For this review, take the finished solid that the model builds, in its own axes (mm). Round coordinates to 2 decimals unless told otherwise and drop trailing zeros. Loops run counter-clockwise (first coordinate to the right, second up) from the corner with the lowest first, then second, coordinate; pieces in that order, holes last. Notation, with made-up numbers: (88.25, -28.75) -> (106.25, -28.75) arc R19 ccw to (106.25, -13.75) -> close; hole circle Ø2 at (21, 61.5). An arc over 180 degrees is marked (long way). One line per question, with ' | ' between items. Start each with the question number.
1. Consider section C-C (y = -9). Write out the cut boundary in (x, z) (3 decimals).
2. Wall thickness on line 1 along X through (y, z) = (-5.75, 9.5); line 2 along Z through (x, y) = (-19.5, -0.5); line 3 along X through (y, z) = (-2.75, 5.5): over which ranges is each line inside the solid? List them lowest first.
3. For pin 1 Ø5 at (x, y) = (20.5, -8.5) entering from -Z, flat-tipped, find the tip position at first contact; note if it passes through.
4. Draft analysis for pull direction X (two halves, no side actions). For faces 1 (the face through (14, -4, 19.05)), 2 (the face through (47.722, -5, 9)), 3 (the face through (-25.36, -4.36, 2.69)), 4 (the face through (-23.99, -4.63, 5.66)), state which applies: pulls with the +X half, pulls with the -X half, needs draft (parallel to the pull), parting line crosses it, or undercut.
5. Consider section B-B (x = -21). Write out the cut boundary in (y, z), and give its area (3 significant figures).
6. Consider section A-A (z = 10.5). Write out the cut boundary in (x, y).
7. Consider section D-D (z = 17). Write out the cut boundary in (x, y), and give its area (3 significant figures).
```python
from build123d import *

# Parameters (mm, degrees)
F0_W        = 76.2
F0_H        = 19.05
F1_DEPTH    = 19.05
F3_D        = 12.7
F4_T1_DEPTH = 68.58


# Not quite as in the source:
# - a fillet or chamfer that OpenCascade refuses, or shapes differently, is made with other operations: its cross-section is extruded or revolved along the edge and cut away or added


with BuildPart() as f1:
    # F0 (on Top) → F1 (new body)
    with BuildSketch(Plane.XY):
        with Locations((9.6218887268, -4.4917178258)):
            Rectangle(F0_W, F0_H)
    extrude(amount=F1_DEPTH)

    # F3 (through all)
    with Locations(Plane(origin=(0, 5.0332821742, 0), x_dir=(-1, 0, 0), z_dir=(0, 1, 0))):
        with Locations((18.9531112732, 9.525)):
            Hole(F3_D / 2)

    # F4: fillet of radius 9.906 on 2 edges, made by hand

    # F4_s2 → F4_t1 (cut)
    with BuildSketch(Plane.XZ.offset(-29.7982821742)):
        with BuildLine():
            ThreePointArc((-18.5721112732, 19.05), (-25.5767110476, 16.1485997744), (-28.4781112732, 9.144))
            Line((-28.4781112732, 9.144), (-28.4781112732, 19.05))
            Line((-28.4781112732, 19.05), (-18.5721112732, 19.05))
        make_face()
        with BuildLine():
            ThreePointArc((-18.5721112732, 0), (-25.5767110476, 2.9014002256), (-28.4781112732, 9.906))
            Line((-28.4781112732, 9.906), (-28.4781112732, 0))
            Line((-28.4781112732, 0), (-18.5721112732, 0))
        make_face()
    extrude(amount=F4_T1_DEPTH, mode=Mode.SUBTRACT)


solid = f1.part
```
Answer block:
1) outline: (-28.471, 9.525) arc R9.906 ccw to (-18.572, 0) -> (47.722, 0) -> (47.722, 19.05) -> (-18.572, 19.05) arc R9.906 ccw to start; hole circle Ø12.7 at (-18.953, 9.525)
2) line 1: x = -28.47 to -25.3, -12.6 to 47.72 | line 2: z = 0.04 to 3.2, 15.85 to 19.01 | line 3: x = -27.44 to -23.86, -14.04 to 47.72
3) pin 1: stops at z = 0
4) face 1: needs draft | face 2: pulls with the +X half | face 3: pulls with the -X half | face 4: undercut
5) outline: (-14.02, 0.3) -> (5.03, 0.3) -> (5.03, 3.51) -> (-14.02, 3.51) -> close; (-14.02, 15.54) -> (5.03, 15.54) -> (5.03, 18.75) -> (-14.02, 18.75) -> close | area: 122 mm2
6) outline: (-28.38, -14.02) -> (-25.23, -14.02) -> (-25.23, 5.03) -> (-28.38, 5.03) -> close; (-12.68, -14.02) -> (47.72, -14.02) -> (47.72, 5.03) -> (-12.68, 5.03) -> close
7) outline: (-24.61, -14.02) -> (47.72, -14.02) -> (47.72, 5.03) -> (-24.61, 5.03) -> close | area: 1,380 mm2
